The listing builds one solid part. Answer for the finished solid, in the listing's coordinates (mm). A direction names the side the tool comes from. Give positions to 0.01 mm unless a question says otherwise; leave off trailing zeros. Write each loop counter-clockwise with the first axis right and the second up, starting at its lowest first coordinate (ties: lowest second). Pieces come first, ordered by that corner, then holes. Notation, with made-up numbers: (31, 57) - (65, 57) arc R12 ccw to (65, 72) - close; hole circle Ø5 at (41.25, 29.25). An arc over 180 degrees is marked (long way). Return JSON: item names as keys, results as strings.
from build123d import *

# Parameters (mm, degrees)
F1_DEPTH = 500
F2_T     = -2


with BuildPart() as f1:
    # F0 (on Front) → F1 (new body)
    with BuildSketch(Plane.XZ):
        Polygon((60, 70), (-60, 70), (-60, 20), (0, 0), (60, 20), align=None)
    extrude(amount=F1_DEPTH)

    # F2
    f2_openings = [f1.faces().sort_by_distance(p)[0] for p in [
        (0, -250, 70),
        (0, -500, 39.722222),
        (0, 0, 39.722222),
    ]]
    offset(amount=F2_T, openings=f2_openings)


solid = f1.part
Item 1: Consider L1, parallel to X at y = -468, z = 51; L2, parallel to Z at x = 18, y = -391; L3, parallel to Z at x = -2.5, y = -398.5. Determine where each line is inside the solid, lowest interval first.
Answer below:
{"L1": "x = -60 to -58, 58 to 60", "L2": "z = 6 to 8.11", "L3": "z = 0.83 to 2.94"}
Item 2: A cutting plane is placed at D-D on z = 7. Determine the outline of the cut face in (x, y).
Answer below:
{"outline": "(-21, -500) - (-14.68, -500) - (-14.68, 0) - (-21, 0) - close; (14.68, -500) - (21, -500) - (21, 0) - (14.68, 0) - close"}
Item 3: A cutting plane is placed at A-A on z = 34.5. Determine the outline of the cut face in (x, y), then the cut area to 3 significant figures.
Answer below:
{"outline": "(-60, -500) - (-58, -500) - (-58, 0) - (-60, 0) - close; (58, -500) - (60, -500) - (60, 0) - (58, 0) - close", "area": "2,000 mm²"}
Item 4: The mould has two halves that part along X. Classify faces 3 (the face through (-31, 0, 12)), 4 (the face through (-60, -246, 45)), 5 (the face through (28.59, -246.5, 11.64)): +X half, -X half, draft (parallel to the pull), parting line (faces both ways), or undercut.
Answer below:
{"face 3": "draft", "face 4": "-X half", "face 5": "undercut"}
Item 5: A cutting plane is placed at C-C on x = -8. Determine the outline of the cut face in (y, z).
Answer below:
{"outline": "(-500, 2.67) - (0, 2.67) - (0, 4.77) - (-500, 4.77) - close"}
Item 6: Flat-ended cylindrical pins translate along their axes: P1, Ø5, axis at x = 26.5, y = -209.5, coming from the +Z side; P2, Ø10, axis at x = -26.5, y = -334.5, coming from the -Z side. Find the tip coordinate at first contact, or state that the pin passes through.
Answer below:
{"P1": "stops at z = 11.77", "P2": "stops at z = 7.17"}
Item 7: For faces 1 (the face through (60, -246, 45)), 2 (the face through (-29.41, -246.5, 11.91)), determine the directions among +Z, -Z, +X, -X, +Y, -Y from which every point of the face is accessible in a straight line to the end or side of a thin tool.
Answer below:
{"face 1": "+Z, -Z, +X, +Y, -Y", "face 2": "+Z, +Y, -Y"}
Item 8: A cutting plane is placed at B-B on y = -241. Determine the outline of the cut face in (x, z).
Answer below:
{"outline": "(-60, 20) - (0, 0) - (60, 20) - (60, 70) - (58, 70) - (58, 21.44) - (0, 2.11) - (-58, 21.44) - (-58, 70) - (-60, 70) - close"}
